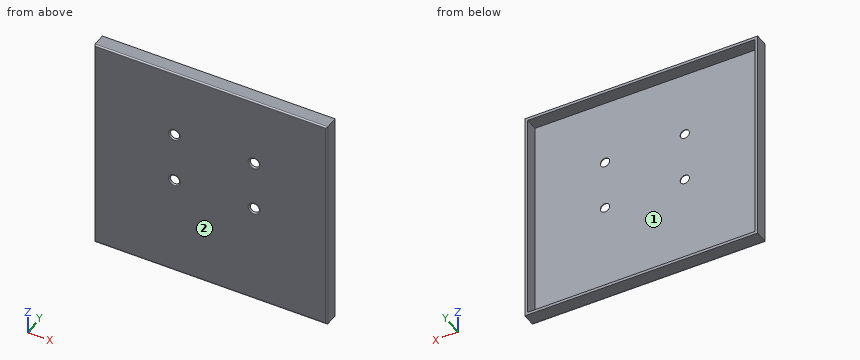
```python
from build123d import *

# Parameters (mm, degrees)
SKETCH1_W           = 164
SKETCH1_H           = 154
SKETCH1_R           = 3.25
BOSS_EXTRUDE1_DEPTH = 10
SKETCH2_W           = 160
SKETCH2_H           = 150
CUT_EXTRUDE1_DEPTH  = 9
FILLET2_R           = 1


with BuildPart() as part:
    # Sketch1 → Boss-Extrude1 (new body)
    with BuildSketch(Plane(origin=(0, 0, 0), x_dir=(1, 0, 0), z_dir=(0, 1, 0))):
        with Locations((-30.679775281, -51.803370787)):
            Rectangle(SKETCH1_W, SKETCH1_H)
        with Locations(Location((-56.229503417, -45.223629633, 0), (0, 0, 270))):
            Circle(SKETCH1_R, mode=Mode.SUBTRACT)
        with Locations(Location((0, -45.223629633, 0), (0, 0, 270))):
            Circle(SKETCH1_R, mode=Mode.SUBTRACT)
        with Locations(Location((-56.229503417, -80.657592441, 0), (0, 0, 270))):
            Circle(SKETCH1_R, mode=Mode.SUBTRACT)
        with Locations(Location((0, -80.657592441, 0), (0, 0, 270))):
            Circle(SKETCH1_R, mode=Mode.SUBTRACT)
    extrude(amount=BOSS_EXTRUDE1_DEPTH)

    # Sketch2 → Cut-Extrude1 (cut)
    with BuildSketch(Plane(origin=(0, 10, 0), x_dir=(1, 0, 0), z_dir=(0, 1, 0))):
        with Locations((-30.679775281, -51.803370787)):
            Rectangle(SKETCH2_W, SKETCH2_H)
    extrude(amount=-CUT_EXTRUDE1_DEPTH, mode=Mode.SUBTRACT)

    # Fillet2
    fillet2_edges = [part.edges().sort_by_distance(p)[0] for p in [
        (-56.229503417, 0, 41.973629633),
        (0, 0, 41.973629633),
        (-56.229503417, 0, 77.407592441),
        (0, 0, 77.407592441),
        (-30.679775281, 0, -25.196629213),
        (51.320224719, 0, 51.803370787),
        (-30.679775281, 0, 128.803370787),
        (-112.679775281, 0, 51.803370787),
    ]]
    fillet(fillet2_edges, radius=FILLET2_R - 0.0001)  # a hair under: the kernel refuses the full size


solid = part.part
```
Here's how the part is built. I have some questions about the finished solid (model axes, mm). Face numbers are marked on the shaded views. Round coordinates to 2 decimals unless told otherwise and drop trailing zeros. Order: outer loops, then holes, each group sorted by start corner. A loop starts at its lowest first (then second) coordinate and runs counter-clockwise, first axis right, second up. Notation, with made-up numbers: M -6.75,56.5 L 14.25,56.5 A30 ccw 14.25,82.5 Z; hole C 70,47 d3. An arc over 180 degrees is marked long. One line per question, with ' | ' between items.
1) I want a section at A-A, the plane x = 0. State how many separate pieces and enclosed holes the cut face has, then the cut area to 3 significant figures.
Working result:
separate pieces: 3 | enclosed holes: 0 | area: 176 mm²
2) I want a section at B-B, the plane y = 7.5. Write out the boundary of the cut face in (x, z).
Working result:
outline: M -112.68,-25.2 L 51.32,-25.2 L 51.32,128.8 L -112.68,128.8 Z; hole M -110.68,-23.2 L 49.32,-23.2 L 49.32,126.8 L -110.68,126.8 Z
3) If we mould it in two halves opening along Z, with no side actions, what happens to the marked faces 1 and 2? For each: +Z half, -Z half, draft (parallel to the pull), parting line (faces both ways), or undercut.
Working result:
face 1: undercut | face 2: draft
4) I need wall thicknesses on line 1 along X through (y, z) = (1.25, 53.5); line 2 along Z through (x, y) = (0, 1.05); line 3 along Y through (x, z) = (-79.5, 13). Which ranges of each line are inside material? Lowest first, please.
Working result:
line 1: -112.68 to -110.68, 49.32 to 51.32 | line 2: -25.2 to -23.2, 126.8 to 128.8 | line 3: 0 to 1
5) I want a section at C-C, the plane z = -2. Write out the boundary of the cut face in (x, y).
Working result:
outline: M -112.68,1 A1 ccw -111.68,0 L 50.32,0 A1 ccw 51.32,1 L 51.32,10 L 49.32,10 L 49.32,1 L -110.68,1 L -110.68,10 L -112.68,10 Z
6) For pin 1 Ø7.5 at (x, z) = (0, 80.66) entering from +Y, with a flat end and sliding along its axis, tell me the tip position at first contact or that it passes through.
Working result:
pin 1: y = 1
